```python
from build123d import *

# Parameters (mm, degrees)
SKETCH_W        = 27
SKETCH_H        = 75
PAD_DEPTH       = 10
SKETCH001_W     = 27
SKETCH001_H     = 10
PAD001_DEPTH    = 0.4
POCKET_DEPTH    = 5
SKETCH011_W     = 14.5
SKETCH011_H     = 0.4
PAD004_DEPTH    = 0.4
SKETCH012_R     = 2.5
PAD005_DEPTH    = 10.4
SKETCH009_R     = 1.5
POCKET001_DEPTH = 10.401
FILLET_R        = 2


with BuildPart() as part:
    # Sketch → Pad (new body)
    with BuildSketch(Plane.XY):
        Polygon((0, 0), (15.5, 0), (15.5, 39.5), (15.5, 79), (0, 79), (-15.5, 79), (-15.5, 39.5), (-15.5, 0), align=None)
        with Locations((0, 39.5)):
            Rectangle(SKETCH_W, SKETCH_H, mode=Mode.SUBTRACT)
    extrude(amount=PAD_DEPTH)

    # Sketch001 → Pad001 (join)
    with BuildSketch(Plane.XY):
        Polygon((-15.5, 79), (-15.5, 39.5), (-15.5, 0), (0, 0), (15.5, 0), (15.5, 39.5), (15.5, 79), (0, 79), align=None)
        with Locations((0, 7)):
            Rectangle(SKETCH001_W, SKETCH001_H, mode=Mode.SUBTRACT)
    extrude(amount=-PAD001_DEPTH)

    # Sketch010 (on DatumPlane) → Pocket (cut)
    with BuildSketch(Plane(origin=(0, 0, 10), x_dir=(-1, 0, 0), z_dir=(0, 0, 1))):
        Polygon((0, 0), (7.25, 0), (7.25, -2), (-7.25, -2), (-7.25, 0), align=None)
    extrude(amount=-POCKET_DEPTH, mode=Mode.SUBTRACT)

    # Sketch011 (on DatumPlane) → Pad004 (join)
    with BuildSketch(Plane(origin=(0, 0, 5), x_dir=(-1, 0, 0), z_dir=(0, 0, 1))):
        with Locations((0, -0.6)):
            Rectangle(SKETCH011_W, SKETCH011_H)
    extrude(amount=PAD004_DEPTH)

    # Sketch012 (on DatumPlane) → Pad005 (join)
    with BuildSketch(Plane(origin=(-15.5, 39.5, 10), x_dir=(-1, 0, 0), z_dir=(0, 0, 1))):
        with Locations((-2.5, 24.5)):
            Circle(SKETCH012_R)
        with Locations((-28.5, 24.5)):
            Circle(SKETCH012_R)
        with Locations((-28.5, -24.5)):
            Circle(SKETCH012_R)
        with Locations((-2.5, -24.5)):
            Circle(SKETCH012_R)
    extrude(amount=-PAD005_DEPTH)

    # Sketch009 (on DatumPlane) → Pocket001 (cut, through all)
    with BuildSketch(Plane(origin=(-15.5, 39.5, 10), x_dir=(-1, 0, 0), z_dir=(0, 0, 1))):
        with Locations((-28.5, 24.5)):
            Circle(SKETCH009_R)
        with Locations((-2.5, 24.5)):
            Circle(SKETCH009_R)
        with Locations((-28.5, -24.5)):
            Circle(SKETCH009_R)
        with Locations((-2.5, -24.5)):
            Circle(SKETCH009_R)
    extrude(amount=-POCKET001_DEPTH, mode=Mode.SUBTRACT)

    # Fillet
    fillet_edges = [part.edges().sort_by_distance(p)[0] for p in [
        (-15.5, 0, 5),
        (15.5, 0, 5),
        (15.5, 79, 5),
        (-15.5, 79, 5),
    ]]
    fillet(fillet_edges, radius=FILLET_R)


solid = part.part
```
Check sheet for the modelled part. Datum: model origin and axes. Units: mm. A direction names the side the tool comes from. Round coordinates to 2 decimals unless told otherwise and drop trailing zeros. Order: outer loops, then holes, each group sorted by start corner. A loop starts at its lowest first (then second) coordinate and runs counter-clockwise, first axis right, second up. Notation, with made-up numbers: (62, 6) - (97, 6) arc R11 cw to (97, 22) - close; hole circle Ø11 at (68, 34). An arc over 180 degrees is marked (long way). Answer as CSV lines item,"result". Start each with the question number.
1) Draft check along X on faces 1 (the face through (-14, 43, 10)), 2 (the face through (-7.25, 1, 8)), 3 (the face through (15.5, 39, 5)). Enter one of: +X half, -X half, draft (parallel to the pull), parting line (faces both ways), or undercut.
2) Section check C-C (z = 3.25). Record the cut outline in (x, y).
3) Depth check by flat-ended pin: pin 1 (2.5 mm diameter, centred on x = -13, y = 15, fed in from +Z); pin 2 (8 mm diameter, centred on x = -3, y = 44, fed in from +Z); pin 3 (0.6 mm diameter, centred on x = 1.5, y = 1, fed in from +Z). Enter the tip coordinate at first touch or a pass-through.
4) Section check D-D (z = 8.5). Record the cut outline in (x, y).
5) Section check B-B (y = 15). Record the cut outline in (x, z), then the cut area to 3 significant figures.
6) Scan lines: probe 1 along X at (y, z) = (15, 7.5); probe 2 along Y at (x, z) = (-11, 7.75); probe 3 along Y at (x, z) = (13, 7.75). Record each from-to range of solid material in increasing order.
7) Tool access check on faces 4 (the face through (0, 45, 0)), 5 (the face through (0, 2, 4)), 6 (the face through (-15.5, 40, 5)). Record the directions out of +Z, -Z, +X, -X, +Y, -Y that give a thin tool (end or side, any length) a straight path to the whole face; none if there is none.
8) Section check A-A (x = -9). Record the cut outline in (y, z).
Determined:
1,face 1,"draft"
1,face 2,"undercut"
1,face 3,"+X half"
2,outline,"(-15.5, 2) arc R2 ccw to (-13.5, 0) - (13.5, 0) arc R2 ccw to (15.5, 2) - (15.5, 77) arc R2 ccw to (13.5, 79) - (-13.5, 79) arc R2 ccw to (-15.5, 77) - close; hole circle Ø3 at (-13, 15); hole circle Ø3 at (-13, 64); hole (-13.5, 2) - (13.5, 2) - (13.5, 12.55) arc R2.5 cw (long way) to (13.5, 17.45) - (13.5, 61.55) arc R2.5 cw (long way) to (13.5, 66.45) - (13.5, 77) - (-13.5, 77) - (-13.5, 66.45) arc R2.5 cw (long way) to (-13.5, 61.55) - (-13.5, 17.45) arc R2.5 cw (long way) to (-13.5, 12.55) - close; hole circle Ø3 at (13, 15); hole circle Ø3 at (13, 64)"
3,pin 1,"through"
3,pin 2,"z = 0"
3,pin 3,"z = 5.4"
4,outline,"(-15.5, 2) arc R2 ccw to (-13.5, 0) - (-7.25, 0) - (-7.25, 2) - (-13.5, 2) - (-13.5, 12.55) arc R2.5 ccw (long way) to (-13.5, 17.45) - (-13.5, 61.55) arc R2.5 ccw (long way) to (-13.5, 66.45) - (-13.5, 77) - (13.5, 77) - (13.5, 66.45) arc R2.5 ccw (long way) to (13.5, 61.55) - (13.5, 17.45) arc R2.5 ccw (long way) to (13.5, 12.55) - (13.5, 2) - (7.25, 2) - (7.25, 0) - (13.5, 0) arc R2 ccw to (15.5, 2) - (15.5, 77) arc R2 ccw to (13.5, 79) - (-13.5, 79) arc R2 ccw to (-15.5, 77) - close; hole circle Ø3 at (-13, 15); hole circle Ø3 at (-13, 64); hole circle Ø3 at (13, 15); hole circle Ø3 at (13, 64)"
5,outline,"(-15.5, -0.4) - (-14.5, -0.4) - (-14.5, 10) - (-15.5, 10) - close; (-11.5, -0.4) - (11.5, -0.4) - (11.5, 10) - (10.5, 10) - (10.5, 0) - (-10.5, 0) - (-10.5, 10) - (-11.5, 10) - close; (14.5, -0.4) - (15.5, -0.4) - (15.5, 10) - (14.5, 10) - close"
5,area,"50.0 mm^2"
6,probe 1,"-15.5 to -14.5, -11.5 to -10.5, 10.5 to 11.5, 14.5 to 15.5"
6,probe 2,"0 to 2, 13.5 to 16.5, 62.5 to 65.5, 77 to 79"
6,probe 3,"0 to 2, 12.5 to 13.5, 16.5 to 17.5, 61.5 to 62.5, 65.5 to 66.5, 77 to 79"
7,face 4,"+Z"
7,face 5,"+Z, -Z"
7,face 6,"+Z, -Z, -X, +Y, -Y"
8,outline,"(0, -0.4) - (2, -0.4) - (2, 10) - (0, 10) - close; (12, -0.4) - (79, -0.4) - (79, 10) - (77, 10) - (77, 0) - (12, 0) - close"
